```python
from build123d import *

# Parameters (mm, degrees)
SKETCH1_R           = 25
BOSS_EXTRUDE1_DEPTH = 7
SKETCH2_R           = 7.5
CUT_EXTRUDE1_DEPTH  = 37.041642582
SKETCH3_R           = 1.922442869
CUT_EXTRUDE2_DEPTH  = 4.826156
CIRPATTERN1_START   = 2.173843947
CIRPATTERN1_DEPTH   = 4.826156053


# Read off the part's stored shape, not the designer's step: CirPattern1
with BuildPart() as part:
    # Sketch1 → Boss-Extrude1 (new body)
    with BuildSketch(Plane(origin=(0, 0, 0), x_dir=(1, 0, 0), z_dir=(0, 1, 0))):
        with Locations(Location((0, 0, 0), (0, 0, 270))):
            Circle(SKETCH1_R)
    extrude(amount=BOSS_EXTRUDE1_DEPTH)

    # Sketch2 → Cut-Extrude1 (cut, through all)
    with BuildSketch(Plane(origin=(0, 0, 0), x_dir=(1, 0, 0), z_dir=(0, 1, 0))):
        with Locations(Location((0, 0, 0), (0, 0, 270))):
            Circle(SKETCH2_R)
    extrude(amount=CUT_EXTRUDE1_DEPTH, mode=Mode.SUBTRACT)

    # Sketch3 → Cut-Extrude2 (cut)
    with BuildSketch(Plane(origin=(0, 7, 0), x_dir=(1, 0, 0), z_dir=(0, 1, 0))):
        with Locations((-6.922121964, 0)):
            Circle(SKETCH3_R)
    extrude(amount=-CUT_EXTRUDE2_DEPTH, mode=Mode.SUBTRACT)

    # CirPattern1 outline → CirPattern1 (cut)
    with BuildSketch(Plane(origin=(0, 0, 0), x_dir=(1, 0, 0), z_dir=(0, 1, 0)).offset(CIRPATTERN1_START)):
        with BuildLine():
            ThreePointArc((-1.893021822, 7.257166691), (0, 7.5), (1.893021822, 7.257166691))
            ThreePointArc((1.893021822, 7.257166691), (0, 8.844564833), (-1.893021822, 7.257166691))
        make_face()
        with BuildLine():
            ThreePointArc((7.257166691, -1.893021822), (8.844564833, 0), (7.257166691, 1.893021822))
            ThreePointArc((7.257166691, 1.893021822), (7.5, 0), (7.257166691, -1.893021822))
        make_face()
        with BuildLine():
            ThreePointArc((1.893021822, -7.257166691), (0, -7.5), (-1.893021822, -7.257166691))
            ThreePointArc((-1.893021822, -7.257166691), (0, -8.844564833), (1.893021822, -7.257166691))
        make_face()
    extrude(amount=CIRPATTERN1_DEPTH, mode=Mode.SUBTRACT)


solid = part.part
```
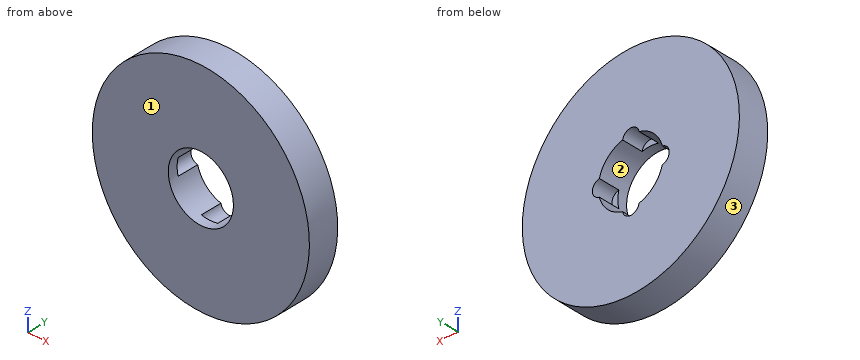
Input: part model. Units: mm. Frame: model coordinates. Face numbers are marked on the shaded views. Give positions to 0.01 mm unless a question says otherwise; leave off trailing zeros. Order: outer loops, then holes, each group sorted by start corner. A loop starts at its lowest first (then second) coordinate and runs counter-clockwise, first axis right, second up.
1. Draft query along Z for the marked faces 1, 2 and 3. Return one class per face: released by +Z, released by -Z, zero draft, split by the parting line, or undercut.
Computed:
face 1: zero draft
face 2: undercut
face 3: split by the parting line
2. Cut plane D-D (z = 15). Return loops of the section in (x, y), and give its area (3 significant figures).
Computed:
outline: (-20, 0) - (20, 0) - (20, 7) - (-20, 7) - close
area: 280 mm2
3. Pin query (flat end, axial travel): pin 1 Ø12 at (x, z) = (0, 0) entering from -Y; pin 2 Ø6 at (x, z) = (-14.5, -5.5) entering from -Y; pin 3 Ø1.3 at (x, z) = (-8, 0) entering from +Y. Return the tip coordinate at first contact, or that it passes through.
Computed:
pin 1: passes through
pin 2: stops at y = 0
pin 3: stops at y = 2.17
4. Cut plane B-B (z = 0). Return loops of the section in (x, y), and give its area (3 significant figures).
Computed:
outline: (-25, 0) - (-7.5, 0) - (-7.5, 2.17) - (-8.84, 2.17) - (-8.84, 7) - (-25, 7) - close; (7.5, 0) - (25, 0) - (25, 7) - (8.84, 7) - (8.84, 2.17) - (7.5, 2.17) - close
area: 232 mm2
5. Line query: probe 1 along X at (y, z) = (1.75, 0.5) (3 decimals); probe 2 along X at (y, z) = (6.75, 5); probe 3 along Z at (x, y) = (6.5, 6.75). Output: solid intervals per line, ascending.
Computed:
probe 1: x = -24.995 to -7.483, 7.483 to 24.995
probe 2: x = -24.49 to -5.59, 5.59 to 24.49
probe 3: z = -24.14 to -3.74, 3.74 to 24.14
6. Cut plane A-A (x = 0). Return loops of the section in (y, z).
Computed:
outline: (0, -25) - (7, -25) - (7, -8.84) - (2.17, -8.84) - (2.17, -7.5) - (0, -7.5) - close; (0, 7.5) - (2.17, 7.5) - (2.17, 8.84) - (7, 8.84) - (7, 25) - (0, 25) - close
7. Cut plane C-C (y = 1.5). Return loops of the section in (x, z), and give its area (3 significant figures).
Computed:
outline: circle Ø50 at (0, 0); hole circle Ø15 at (0, 0)
area: 1,790 mm2
